Geometry: final body of the model. Coordinates: model frame, mm. Face numbers are marked on the shaded views. A direction names the side the tool comes from. Give positions to 0.01 mm unless a question says otherwise; leave off trailing zeros. Loops run counter-clockwise (first coordinate to the right, second up) from the corner with the lowest first, then second, coordinate; pieces in that order, holes last. Notation, with made-up numbers: (75, 79.25) -> (103, 79.25) arc R18 cw to (103, 92.25) -> close; hole circle Ø5 at (-36, -8). An arc over 180 degrees is marked (long way). Answer in a Markdown table with one row per item. Add a question column.
from build123d import *

# Parameters (mm, degrees)
SKETCH2_R            = 2.5
SKETCH2_R_2          = 2
BOSS_EXTRUDE1_DEPTH  = 7.2
MOVE_FACE1_OUTLINE_R = 2.5
MOVE_FACE1_DEPTH     = 7.2
CUT_EXTRUDE2_DEPTH   = 92.988260121
FILLET1_R            = 2.5
SKETCH5_R            = 2.5
CUT_EXTRUDE3_DEPTH   = 91.271536943
CUT_EXTRUDE4_DEPTH   = 91.271536943
SKETCH8_R            = 4.5
SKETCH8_R_2          = 4
CUT_EXTRUDE5_DEPTH   = 3


# Read off the part's stored shape, not the designer's step: Move Face1
with BuildPart() as part:
    # Sketch2 → Boss-Extrude1 (new body)
    with BuildSketch(Plane.XY):
        with BuildLine():
            Line((3, 4), (-33, 4))
            Line((-33, 4), (-33, -4))
            Line((-33, -4), (3, -4))
            ThreePointArc((3, -4), (5.828427125, -5.171572875), (7, -8))
            Line((7, -8), (7, -12))
            ThreePointArc((7, -12), (5.828427125, -14.828427125), (3, -16))
            Line((3, -16), (-33, -16))
            Line((-33, -16), (-33, -21.632357189))
            ThreePointArc((-33, -21.632357189), (-32.276311449, -25.736598909), (-30.192533317, -29.345808505))
            Line((-30.192533317, -29.345808505), (-17.821439842, -44.089103599))
            ThreePointArc((-17.821439842, -44.089103599), (-16.447735116, -45.143184308), (-14.757262069, -45.51795316))
            Line((-14.757262069, -45.51795316), (14.512756385, -45.51795316))
            ThreePointArc((14.512756385, -45.51795316), (17.34118351, -46.689526036), (18.512756385, -49.51795316))
            Line((18.512756385, -49.51795316), (18.512756385, -81))
            Line((18.512756385, -81), (8.861465874, -81))
            Line((8.861465874, -81), (1.705289702, -81))
            ThreePointArc((1.705289702, -81), (-3.366129439, -79.875693444), (-7.487243615, -76.713451316))
            Line((-7.487243615, -76.713451316), (-40.192533317, -37.736804817))
            ThreePointArc((-40.192533317, -37.736804817), (-42.276311449, -34.12759522), (-43, -30.023353501))
            Line((-43, -30.023353501), (-43, 21))
            Line((-43, 21), (-33, 21))
            Line((-33, 21), (-33, 16))
            Line((-33, 16), (3, 16))
            ThreePointArc((3, 16), (5.828427125, 14.828427125), (7, 12))
            Line((7, 12), (7, 8))
            ThreePointArc((7, 8), (5.828427125, 5.171572875), (3, 4))
        make_face()
        with Locations((0, 10)):
            Circle(SKETCH2_R, mode=Mode.SUBTRACT)
        with Locations(Location((0, -10, 0), (0, 0, 180))):
            Circle(SKETCH2_R, mode=Mode.SUBTRACT)
        with Locations((12.512756385, -51.51795316)):
            Circle(SKETCH2_R_2, mode=Mode.SUBTRACT)
        with Locations((-2.487243615, -72.51795316)):
            Circle(SKETCH2_R_2, mode=Mode.SUBTRACT)
    extrude(amount=BOSS_EXTRUDE1_DEPTH)

    # Move Face1 outline → Move Face1 (cut)
    # profile 1 of 4: a face of its own
    with BuildSketch(Plane.XY):
        with BuildLine():
            Line((-3, -8), (-3, -12))
            ThreePointArc((-3, -12), (-4.171572875, -14.828427125), (-7, -16))
            Line((-7, -16), (3, -16))
            ThreePointArc((3, -16), (5.828427125, -14.828427125), (7, -12))
            Line((7, -12), (7, -8))
            ThreePointArc((7, -8), (5.828427125, -5.171572875), (3, -4))
            Line((3, -4), (-7, -4))
            ThreePointArc((-7, -4), (-4.171572875, -5.171572875), (-3, -8))
        make_face()
        with Locations((0, -10)):
            Circle(MOVE_FACE1_OUTLINE_R, mode=Mode.SUBTRACT)
    # profile 2 of 4: a face of its own
    with BuildSketch(Plane.XY):
        with BuildLine():
            ThreePointArc((-7, 16), (-4.171572875, 14.828427125), (-3, 12))
            Line((-3, 12), (-3, 8))
            ThreePointArc((-3, 8), (-4.171572875, 5.171572875), (-7, 4))
            Line((-7, 4), (3, 4))
            ThreePointArc((3, 4), (5.828427125, 5.171572875), (7, 8))
            Line((7, 8), (7, 12))
            ThreePointArc((7, 12), (5.828427125, 14.828427125), (3, 16))
            Line((3, 16), (-7, 16))
        make_face()
        with Locations((0, 10)):
            Circle(MOVE_FACE1_OUTLINE_R, mode=Mode.SUBTRACT)
    # profile 3 of 4: a face of its own
    with BuildSketch(Plane.XY):
        with Locations((-10, 10)):
            Circle(MOVE_FACE1_OUTLINE_R)
    # profile 4 of 4: a face of its own
    with BuildSketch(Plane.XY):
        with Locations((-10, -10)):
            Circle(MOVE_FACE1_OUTLINE_R)
    extrude(amount=MOVE_FACE1_DEPTH, mode=Mode.SUBTRACT)

    # Sketch4 → Cut-Extrude2 (cut, through all)
    with BuildSketch(Plane.XY.offset(7.2)):
        with BuildLine():
            Line((12.512756385, -57.51795316), (4.039792831, -72.51795316))
            ThreePointArc((4.039792831, -72.51795316), (-0.254865674, -78.651361145), (-7.487243615, -76.713451316))
            Line((-7.487243615, -76.713451316), (-9.608649797, -88.557738574))
            Line((-9.608649797, -88.557738574), (26.411143911, -81.246796091))
            Line((26.411143911, -81.246796091), (26.411143911, -45.51795316))
            Line((26.411143911, -45.51795316), (12.512756385, -45.51795316))
            ThreePointArc((12.512756385, -45.51795316), (18.512756385, -51.51795316), (12.512756385, -57.51795316))
        make_face()
    extrude(amount=-CUT_EXTRUDE2_DEPTH, mode=Mode.SUBTRACT)

    # Fillet1
    fillet1_edges = [part.edges().sort_by_distance(p)[0] for p in [
        (12.512756385, -57.51795316, 3.6),
        (4.039792831, -72.51795316, 3.6),
        (-33, 16, 3.6),
        (-33, 4, 3.6),
        (-33, -4, 3.6),
        (-33, -16, 3.6),
        (-43, 21, 3.6),
        (-33, 21, 3.6),
    ]]
    fillet(fillet1_edges, radius=FILLET1_R - 0.0001)  # a hair under: the kernel refuses the full size

    # Sketch5 → Cut-Extrude3 (cut, through all)
    with BuildSketch(Plane.XY.offset(7.2)):
        with Locations((-38, 10)):
            Circle(SKETCH5_R)
        with Locations((-38, -10)):
            Circle(SKETCH5_R)
    extrude(amount=-CUT_EXTRUDE3_DEPTH, mode=Mode.SUBTRACT)

    # Sketch6 → Cut-Extrude4 (cut, through all)
    with BuildSketch(Plane.XY.offset(7.2)):
        with BuildLine():
            Line((1.008892165, -52.51795316), (-10.912898118, -52.51795316))
            ThreePointArc((-10.912898118, -52.51795316), (-13.631821479, -54.250098375), (-13.211031447, -57.446315989))
            Line((-13.211031447, -57.446315989), (-6.085798343, -65.937838139))
            ThreePointArc((-6.085798343, -65.937838139), (-3.512131749, -66.996795417), (-1.175581436, -65.484947907))
            Line((-1.175581436, -65.484947907), (3.620975743, -56.993425757))
            ThreePointArc((3.620975743, -56.993425757), (3.599878251, -54.005739186), (1.008892165, -52.51795316))
        make_face()
    extrude(amount=-CUT_EXTRUDE4_DEPTH, mode=Mode.SUBTRACT)

    # Sketch8 → Cut-Extrude5 (cut)
    with BuildSketch(Plane.XY.offset(7.2)):
        with Locations((-38, 10)):
            Circle(SKETCH8_R)
        with Locations((-10, 10)):
            Circle(SKETCH8_R)
        with Locations((-38, -10)):
            Circle(SKETCH8_R)
        with Locations((-10, -10)):
            Circle(SKETCH8_R)
        with Locations((12.512756385, -51.51795316)):
            Circle(SKETCH8_R_2)
        with Locations((-2.487243615, -72.51795316)):
            Circle(SKETCH8_R_2)
    extrude(amount=-CUT_EXTRUDE5_DEPTH, mode=Mode.SUBTRACT)


solid = part.part
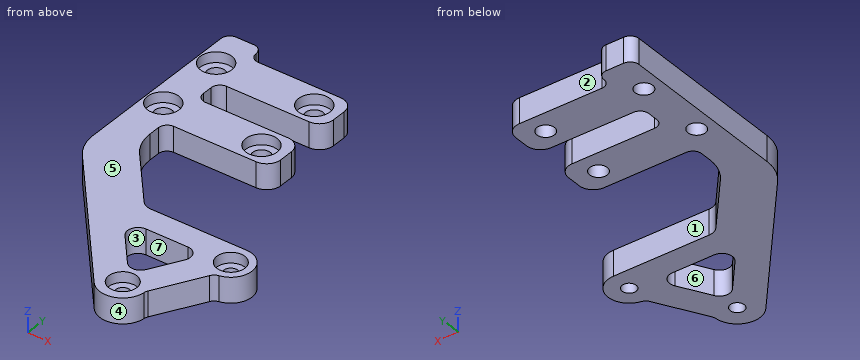
(1) Reachability of the marked faces 1, 2 and 3 from +Z, -Z, +X, -X, +Y, -Y: full face, straight path, thin tool, end or side. Return the list, or none.
(2) Cut plane C-C on z = 1.75. State how many separate pieces and enclosed holes the cut face has, then the cut area to 3 significant figures.
(3) Pin query (flat end, axial travel): pin 1 Ø8 at (x, y) = (-15.5, -38) entering from -Z; pin 2 Ø3 at (x, z) = (-27, 1) entering from -Y; pin 3 Ø1.5 at (x, z) = (-13, 5) entering from -Y; pin 4 Ø2.5 at (y, z) = (-0.5, 2.5) entering from +X. Return the tip coordinate at first contact, or that it passes through.
(4) Cut plane D-D on y = -41.5. Return the cut outline in (x, z), then the cut area to 3 significant figures.
(5) Draft query along Y for the marked faces 4, 5, 6 and 7. Return one class per face: +Y half, -Y half, draft (parallel to the pull), parting line (faces both ways), or undercut.
(6) Cut plane B-B on x = -38.5. Return the cut outline in (y, z).
(7) Cut plane A-A on y = 10. Return the cut outline in (x, z), then the cut area to 3 significant figures.
(8) Material intervals for line 1 along Y through (x, z) = (-17.5, 5.25); line 2 along Y through (x, z) = (-7, 5); line 3 along Y through (x, z) = (-1, 1.75), sorted ascending. Write a range as from..to.
Answer list:
| question | item | result |
|---|---|---|
| 1 | face 1 | +Z, -Z, +X |
| 1 | face 2 | +Z, -Z, +X, +Y |
| 1 | face 3 | +Z, -Z |
| 2 | separate pieces | 1 |
| 2 | enclosed holes | 7 |
| 2 | area | 2,210 mm² |
| 3 | pin 1 | passes through |
| 3 | pin 2 | stops at y = -55.25 |
| 3 | pin 3 | stops at y = -71.04 |
| 3 | pin 4 | stops at x = -32.99 |
| 4 | outline | (-37.03, 0) -> (-19.99, 0) -> (-19.99, 7.2) -> (-37.03, 7.2) -> close |
| 4 | area | 123 mm² |
| 5 | face 4 | -Y half |
| 5 | face 5 | draft |
| 5 | face 6 | undercut |
| 5 | face 7 | undercut |
| 6 | outline | (-39.75, 0) -> (-12.45, 0) -> (-12.45, 4.2) -> (-14.47, 4.2) -> (-14.47, 7.2) -> (-39.75, 7.2) -> close; (-7.55, 0) -> (7.55, 0) -> (7.55, 4.2) -> (5.53, 4.2) -> (5.53, 7.2) -> (-5.53, 7.2) -> (-5.53, 4.2) -> (-7.55, 4.2) -> close; (12.45, 0) -> (21, 0) -> (21, 7.2) -> (14.47, 7.2) -> (14.47, 4.2) -> (12.45, 4.2) -> close |
| 7 | outline | (-43, 0) -> (-40.5, 0) -> (-40.5, 4.2) -> (-42.5, 4.2) -> (-42.5, 7.2) -> (-43, 7.2) -> close; (-35.5, 0) -> (-12.5, 0) -> (-12.5, 4.2) -> (-14.5, 4.2) -> (-14.5, 7.2) -> (-33.5, 7.2) -> (-33.5, 4.2) -> (-35.5, 4.2) -> close; (-7.5, 0) -> (-3, 0) -> (-3, 7.2) -> (-5.5, 7.2) -> (-5.5, 4.2) -> (-7.5, 4.2) -> close |
| 7 | area | 192 mm² |
| 8 | line 1 | y = -64.78..-44.43, -16..-4, 4..16 |
| 8 | line 2 | y = -77.23..-64.85, -52.52..-45.52, -16..-13.35, -6.65..-4, 4..6.65, 13.35..16 |
| 8 | line 3 | y = -78.87..-73.86, -71.18..-65.17, -52.52..-45.52 |
